Answer from the drawing. Dimensions are ordinates in mm from the lowest x, y and z of the part. A direction names the side the tool comes from. Give positions to 0.01 mm unless a question says otherwise; leave off trailing zeros. Order: outer loops, then holes, each group sorted by start corner. A loop starts at its lowest first (then second) coordinate and runs counter-clockwise, first axis right, second up. Notation, with made-up numbers: (80.5, 62) - (123.5, 62) arc R19 cw to (123.5, 87) - close; hole circle Ø11 at (-13, -28.75). An arc over 180 degrees is marked (long way). Answer in a Markdown table with one row per item.
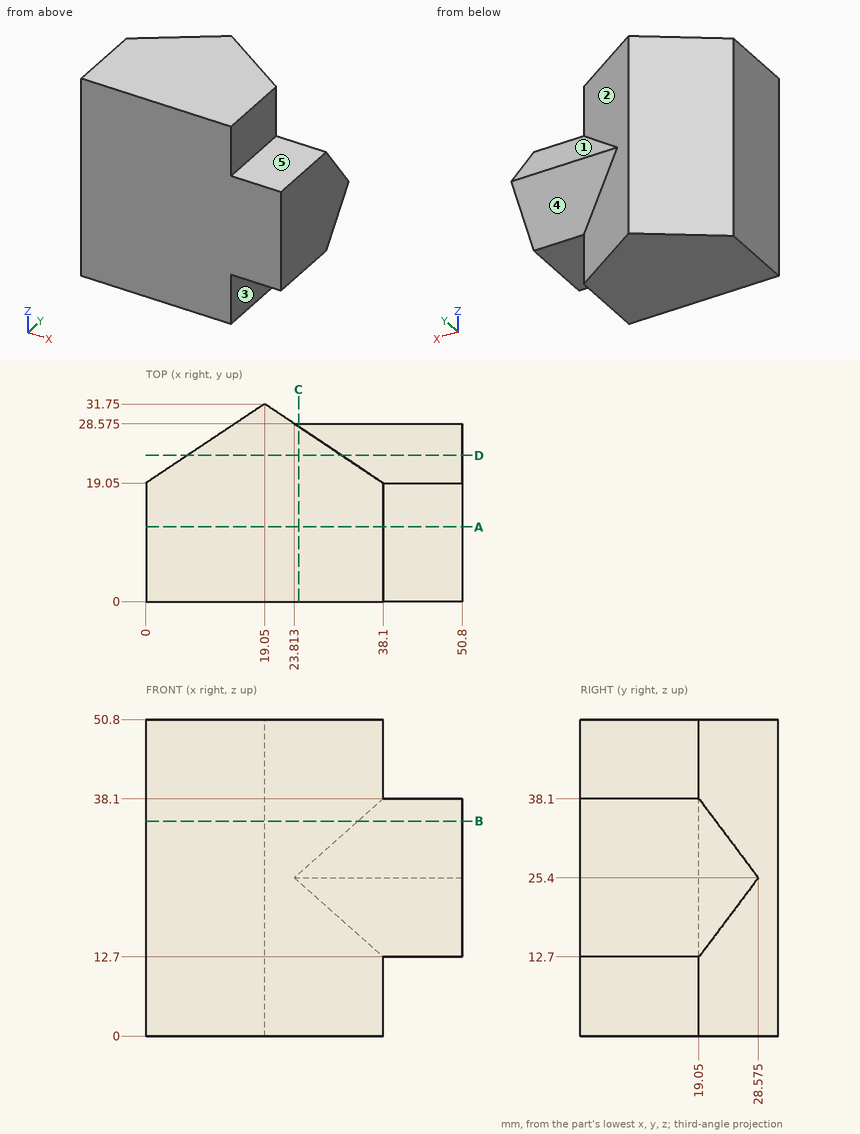
Item 1: Find section C-C on x = 24.5. Write down the section's boundary in (y, z) (1 decimal).
Answer block:
| item | result |
|---|---|
| outline | (0, 0) - (28.1, 0) - (28.1, 24.8) - (28.6, 25.4) - (28.1, 26) - (28.1, 50.8) - (0, 50.8) - close |
Item 2: Which of the six approach directions +Z, -Z, +X, -X, +Y, -Y give full straight-line access (tool end or side, diameter ignored) to the marked faces 1, 2, 3, 4 and 5?
Answer block:
| item | result |
|---|---|
| face 1 | +Z, +X, +Y |
| face 2 | +X, +Y |
| face 3 | -Z, +X, +Y, -Y |
| face 4 | -Z, +X, +Y |
| face 5 | +Z, +X, +Y, -Y |
Item 3: Consider line 1 (Y direction, x = 9.5, z = 2) (1 decimal); line 2 (X direction, y = 18, z = 10); line 3 (Y direction, x = 11, z = 40) (1 decimal). Determine where each line is inside the solid, lowest interval first.
Answer block:
| item | result |
|---|---|
| line 1 | 0 to 25.4 |
| line 2 | 0 to 38.1 |
| line 3 | 0 to 26.4 |
Item 4: Find section B-B on z = 34.5. Write down the section's boundary in (x, y).
Answer block:
| item | result |
|---|---|
| outline | (0, 0) - (50.8, 0) - (50.8, 21.75) - (34.05, 21.75) - (19.05, 31.75) - (0, 19.05) - close |
Item 5: Find section A-A on y = 12. Write down the section's boundary in (x, z), then the cut area to 3 significant figures.
Answer block:
| item | result |
|---|---|
| outline | (0, 0) - (38.1, 0) - (38.1, 12.7) - (50.8, 12.7) - (50.8, 38.1) - (38.1, 38.1) - (38.1, 50.8) - (0, 50.8) - close |
| area | 2,260 mm² |
Item 6: Find section D-D on y = 23.5. Write down the section's boundary in (x, z) (1 decimal).
Answer block:
| item | result |
|---|---|
| outline | (6.7, 0) - (31.4, 0) - (31.4, 18.6) - (50.8, 18.6) - (50.8, 32.2) - (31.4, 32.2) - (31.4, 50.8) - (6.7, 50.8) - close |
Item 7: Each of these flat-tipped pins is pushed along its axis until it touches: P1, Ø4, axis at x = 42.5, y = 6, coming from the +Z side; P2, Ø4, axis at y = 13.5, z = 46, coming from the +X side; P3, Ø10, axis at x = 9, z = 34, coming from the +Y side. Where does it stop, or does it pass through?
Answer block:
| item | result |
|---|---|
| P1 | z = 38.1 |
| P2 | x = 38.1 |
| P3 | y = 28.38 |
